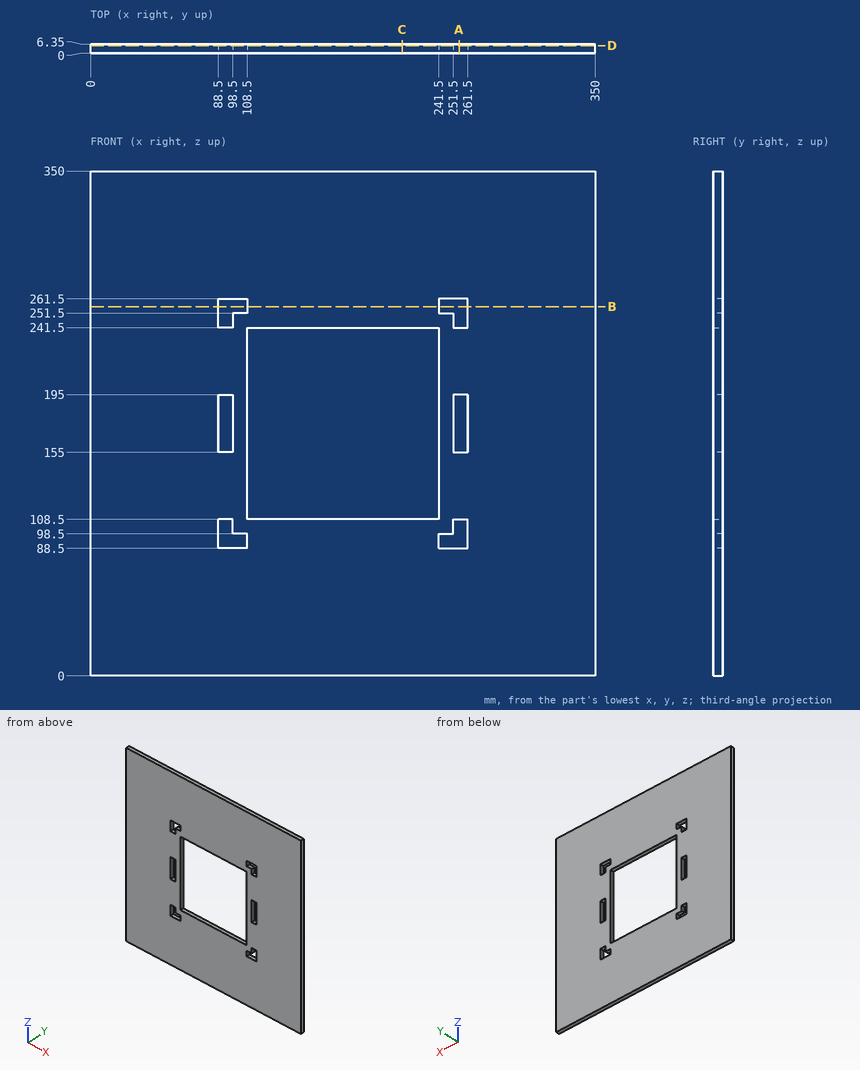
Source: three-view drawing plus pictorial views. Frame: mm from the lowest corner of the part. Coordinates: 2 decimals unless noted, no trailing zeros. Loops run counter-clockwise (first coordinate to the right, second up) from the corner with the lowest first, then second, coordinate; pieces in that order, holes last. Notation, with made-up numbers: (3.5, 49.5) -> (21.5, 49.5) arc R23 cw to (21.5, 75.5) -> close; hole circle Ø8 at (-10.75, 1). An arc over 180 degrees is marked (long way). Answer in a Markdown table with one row per item. Add a question column.
Q1. Section A-A on x = 255.5. Return the cut outline in (y, z).
Q2. Section D-D on y = 5.25. Give the number of separate pieces and of enclosed holes in the cut face, and give its area (3 significant figures).
Q3. Section B-B on z = 256. Return the cut outline in (x, y), and give its area (3 significant figures).
Q4. Section C-C on x = 216. Return the cut outline in (y, z).
Q5. Ray query, line 1 along X through (y, z) = (6.25, 177); line 2 along X through (y, z) = (2, 255.5); line 3 along Z through (x, y) = (90, 0.75). Return the intervals inside material, ascending.
Computed values:
| question | item | result |
|---|---|---|
| 1 | outline | (0, 0) -> (6.35, 0) -> (6.35, 88.5) -> (0, 88.5) -> close; (0, 108.5) -> (6.35, 108.5) -> (6.35, 155) -> (0, 155) -> close; (0, 195) -> (6.35, 195) -> (6.35, 241.5) -> (0, 241.5) -> close; (0, 261.5) -> (6.35, 261.5) -> (6.35, 350) -> (0, 350) -> close |
| 2 | separate pieces | 1 |
| 2 | enclosed holes | 7 |
| 2 | area | 103,000 mm^2 |
| 3 | outline | (0, 0) -> (88.5, 0) -> (88.5, 6.35) -> (0, 6.35) -> close; (108.5, 0) -> (241.5, 0) -> (241.5, 6.35) -> (108.5, 6.35) -> close; (261.5, 0) -> (350, 0) -> (350, 6.35) -> (261.5, 6.35) -> close |
| 3 | area | 1,970 mm^2 |
| 4 | outline | (0, 0) -> (6.35, 0) -> (6.35, 108.5) -> (0, 108.5) -> close; (0, 241.5) -> (6.35, 241.5) -> (6.35, 350) -> (0, 350) -> close |
| 5 | line 1 | x = 0 to 88.5, 98.5 to 108.5, 241.5 to 251.5, 261.5 to 350 |
| 5 | line 2 | x = 0 to 88.5, 108.5 to 241.5, 261.5 to 350 |
| 5 | line 3 | z = 0 to 88.5, 108.5 to 155, 195 to 241.5, 261.5 to 350 |
